Geometry check sheet. Reference: drawing and pictorial views, mm from the part's lowest x, y, z. Coordinates: 2 decimals unless noted, no trailing zeros. Loops run counter-clockwise (first coordinate to the right, second up) from the corner with the lowest first, then second, coordinate; pieces in that order, holes last. Notation, with made-up numbers: (-12, 59.25) -> (20, 59.25) arc R21 ccw to (20, 82.25) -> close; hole circle Ø1 at (-39, 57.25). An arc over 180 degrees is marked (long way). Use one line per item in the form item = value.
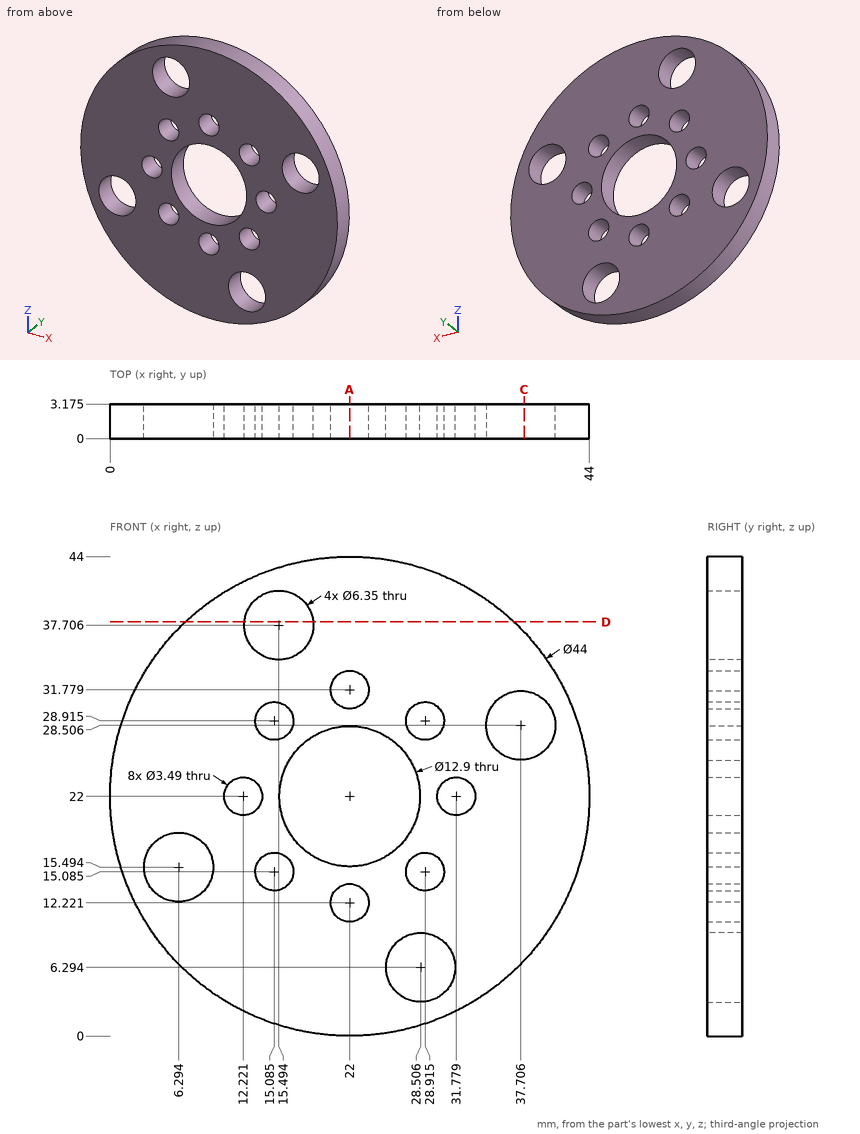
(1) Section check A-A, the plane x = 22. Give the number of separate pieces and of enclosed holes in the cut face.
Established:
separate_pieces = 4
enclosed_holes = 0
(2) Section check D-D, the plane z = 38. Record the boundary of the cut face in (x, y) (1 decimal).
Established:
outline = (6.9, 0) -> (12.3, 0) -> (12.3, 3.2) -> (6.9, 3.2) -> close; (18.7, 0) -> (37.1, 0) -> (37.1, 3.2) -> (18.7, 3.2) -> close
(3) Go/stop test with a flat-tipped pin: P1, Ø1.5, axis at y = 2, z = 28, coming from the +X side (1 decimal). Record where the tip stops, or that it passes through.
Established:
P1 = 43.4
(4) Scan lines: line 1 along Z through (x, y) = (13, 0.6) (1 decimal); line 2 along Z through (x, y) = (19.5, 2.85) (1 decimal); line 3 along X through (y, z) = (1.8, 5.5). Record each from-to range of solid material in increasing order.
Established:
line_1 = 1.9 to 20.4, 23.6 to 35.7, 39.7 to 42.1
line_2 = 0.1 to 16.1, 27.9 to 43.9
line_3 = 7.45 to 25.43, 31.58 to 36.55
(5) Section check C-C, the plane x = 38. Record the boundary of the cut face in (y, z) (1 decimal).
Established:
outline = (0, 6.9) -> (3.2, 6.9) -> (3.2, 25.3) -> (0, 25.3) -> close; (0, 31.7) -> (3.2, 31.7) -> (3.2, 37.1) -> (0, 37.1) -> close
